Build history of the part. All positions in model axes, mm. Face numbers are marked on the shaded views. A direction names the side the tool comes from. Give positions to 0.01 mm unless a question says otherwise; leave off trailing zeros. Loops run counter-clockwise (first coordinate to the right, second up) from the corner with the lowest first, then second, coordinate; pieces in that order, holes last. Notation, with made-up numbers: (8, 43) -> (59, 43) arc R12 cw to (59, 61) -> close; hole circle Ø5 at (31, 55). An arc over 180 degrees is marked (long way). Answer as a JSON object with one key per item and string values. Group by question number.
Q1. Band-saw the part on B-B, the plane y = 0. Write the cut outline in (x, z).
Q2. Band-saw the part on D-D, the plane z = 3.5. Write the cut outline in (x, y), plus the area to 3 significant figures.
Q3. Tool access for the marked faces 1 and 2: list every direction of +Z, -Z, +X, -X, +Y, -Y with a clear straight run to the whole face (end or side of a thin tool).
Q4. Wall check: probe 1 along Z at (x, y) = (-22, -1.5); probe 2 along Z at (x, y) = (-37.25, 0); probe 3 along X at (y, z) = (3.5, 3.5). Give the ranges that are in metal, low to high. Write a range as from..to.
Q5. Band-saw the part on C-C, the plane x = -13.5. Write the cut outline in (y, z), plus the area to 3 significant figures.
Q6. Two-plate mould, pull along Z, no slides. Class the marked faces 3, 4, 5 and 6: pulls with the +Z half, pulls with the -Z half, needs draft (parallel to the pull), parting line crosses it, or undercut.
Q7. Band-saw the part on A-A, the plane z = 10. Write the cut outline in (x, y).
Q8. Drop flat-ended pins along their axis: pin 1 (2 mm diameter, centred on y = -2.5, z = 9, fed in from +X); pin 2 (6 mm diameter, centred on x = -10.5, y = -5, fed in from -Z); pin 3 (3.5 mm diameter, centred on y = 0, z = 10, fed in from -X); pin 4 (4 mm diameter, centred on x = -9.5, z = 14.5, fed in from -Y). Give the stop position or say it passes through.
from build123d import *

# Parameters (mm, degrees)
PAD_DEPTH       = 20
PAD001_DEPTH    = 12
SKETCH002_R     = 1.6
POCKET_DEPTH    = 3.5
SKETCH003_W     = 8
SKETCH003_H     = 9.5
POCKET001_DEPTH = 1.5
PAD002_DEPTH    = 20
SKETCH005_W     = 39.25
SKETCH005_H     = 16
POCKET002_DEPTH = 10
POCKET003_DEPTH = 2


with BuildPart() as part:
    # Sketch → Pad (new body)
    with BuildSketch(Plane.XY):
        Polygon((-36.25, -6), (-38.25, -6), (-38.25, 6), (38.25, 6), (38.25, -6), (36.25, -6), (36.25, 4), (-36.25, 4), align=None)
    extrude(amount=PAD_DEPTH)

    # Sketch001 (on Face1 of Pad) → Pad001 (join)
    with BuildSketch(Plane.XZ.offset(6)):
        Polygon((-38.25, 5.25), (-38.25, 14.75), (-39.75, 12.95), (-39.75, 7.05), align=None)
    pad001 = extrude(amount=-PAD001_DEPTH)

    # Sketch002 (on Face12 of Pad001) → Pocket (cut)
    with BuildSketch(Plane(origin=(-39.75, 0, 0), x_dir=(0, -1, 0), z_dir=(-1, 0, 0))):
        with Locations((0, 10)):
            Circle(SKETCH002_R)
    pocket = extrude(amount=-POCKET_DEPTH, mode=Mode.SUBTRACT)

    # Sketch003 (on Face13 of Pocket) → Pocket001 (cut)
    with BuildSketch(Plane(origin=(-39.75, 0, 0), x_dir=(0, -1, 0), z_dir=(-1, 0, 0))):
        with Locations((0, 10)):
            Rectangle(SKETCH003_W, SKETCH003_H)
    pocket001 = extrude(amount=-POCKET001_DEPTH, mode=Mode.SUBTRACT)

    # Sketch004 (on Face6 of Pocket001) → Pad002 (join)
    with BuildSketch(Plane(origin=(0, 0, 0), x_dir=(1, 0, 0), z_dir=(0, 0, -1))):
        Polygon((-36.25, -4), (-36.25, 6), (3, -4), align=None)
    pad002 = extrude(amount=-PAD002_DEPTH)

    # Sketch005 (on Face1 of Pad002) → Pocket002 (cut)
    with BuildSketch(Plane.XZ.offset(6)):
        with Locations((-16.625, 10)):
            Rectangle(SKETCH005_W, SKETCH005_H)
    pocket002 = extrude(amount=-POCKET002_DEPTH, mode=Mode.SUBTRACT)

    # Mirrored: Pad001, Pocket, Pocket001, Pad002, Pocket002 across YZ
    add(pad001.mirror(Plane.YZ))
    add(pocket.mirror(Plane.YZ), mode=Mode.SUBTRACT)
    add(pocket001.mirror(Plane.YZ), mode=Mode.SUBTRACT)
    add(pad002.mirror(Plane.YZ))
    add(pocket002.mirror(Plane.YZ), mode=Mode.SUBTRACT)

    # Sketch006 (on Face12 of Mirrored) → Pocket003 (cut)
    with BuildSketch(Plane.XZ.offset(-4)):
        with BuildLine():
            ThreePointArc((-27.5, 15), (-32.5, 10), (-27.5, 5))
            Line((-27.5, 5), (27.5, 5))
            ThreePointArc((27.5, 5), (32.5, 10), (27.5, 15))
            Line((27.5, 15), (-27.5, 15))
        make_face()
    extrude(amount=-POCKET003_DEPTH, mode=Mode.SUBTRACT)


solid = part.part
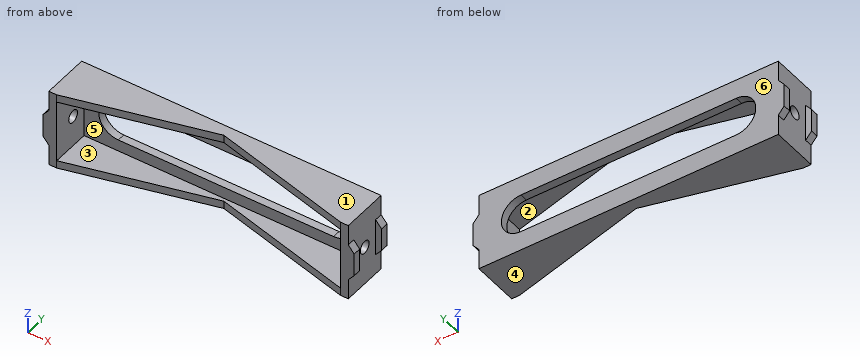
Worked answers:
{
 "1": {"outline": "(-38.25, 0) -> (-12.7, 0) -> (-12.7, 2) -> (-36.25, 2) -> (-36.25, 8.4) -> (-38.25, 8.4) -> close; (-38.25, 11.6) -> (-36.25, 11.6) -> (-36.25, 18) -> (-12.7, 18) -> (-12.7, 20) -> (-38.25, 20) -> close; (12.7, 0) -> (38.25, 0) -> (38.25, 8.4) -> (36.25, 8.4) -> (36.25, 2) -> (12.7, 2) -> close; (12.7, 18) -> (36.25, 18) -> (36.25, 11.6) -> (38.25, 11.6) -> (38.25, 20) -> (12.7, 20) -> close"},
 "2": {"outline": "(-38.25, -6) -> (-36.25, -6) -> (-36.25, 4) -> (36.25, 4) -> (36.25, -6) -> (38.25, -6) -> (38.25, 6) -> (-38.25, 6) -> close", "area": "193 mm2"},
 "3": {"face 1": "+Z, +X, -X, +Y, -Y", "face 2": "-Y"},
 "4": {"probe 1": "0..2, 18..20", "probe 2": "0..8.4, 11.6..20", "probe 3": "-38.25..-36.25, 36.25..38.25"},
 "5": {"outline": "(-0.2, 0) -> (6, 0) -> (6, 5) -> (4, 5) -> (4, 2) -> (-0.2, 2) -> close; (-0.2, 18) -> (4, 18) -> (4, 15) -> (6, 15) -> (6, 20) -> (-0.2, 20) -> close", "area": "36.8 mm2"},
 "6": {"face 3": "undercut", "face 4": "pulls with the -Z half", "face 5": "undercut", "face 6": "needs draft"},
 "7": {"outline": "(-39.75, -6) -> (-36.25, -6) -> (-36.25, -1.6) -> (-38.25, -1.6) -> (-38.25, -4) -> (-39.75, -4) -> close; (-39.75, 4) -> (-38.25, 4) -> (-38.25, 1.6) -> (-36.25, 1.6) -> (-36.25, 4) -> (-32.5, 4) -> (-32.5, 6) -> (-39.75, 6) -> close; (32.5, 4) -> (36.25, 4) -> (36.25, 1.6) -> (38.25, 1.6) -> (38.25, 4) -> (39.75, 4) -> (39.75, 6) -> (32.5, 6) -> close; (36.25, -6) -> (39.75, -6) -> (39.75, -4) -> (38.25, -4) -> (38.25, -1.6) -> (36.25, -1.6) -> close"},
 "8": {"pin 1": "x = 38.25", "pin 2": "through", "pin 3": "x = -38.25", "pin 4": "y = 4"}
}
